```python
from build123d import *

# Parameters (mm, degrees)
SKETCH1_R                 = 31.75
BOSS_EXTRUDE1_DEPTH       = 139
SKETCH3_R                 = 9.5
BOSS_EXTRUDE2_DEPTH       = 2.4
SKETCH3_2_R               = 9.5
BOSS_EXTRUDE3_DEPTH       = 13.75
F_6_32_TAPPED_HOLE1_D     = 2.7051
F_6_32_TAPPED_HOLE1_DEPTH = 9.39
F_6_32_TAPPED_HOLE1_TIP   = 0.81269403
SKETCH7_R                 = 6.25
BOSS_EXTRUDE4_DEPTH       = 2.5
SKETCH7_3_R               = 5
BOSS_EXTRUDE5_DEPTH       = 8.33
SKETCH7_4_R               = 5
BOSS_EXTRUDE6_DEPTH       = 18.5
BOSS_EXTRUDE7_DEPTH       = 0.5


with BuildPart() as part:
    # Sketch1 → Boss-Extrude1 (new, symmetric)
    with BuildSketch(Plane.XY):
        Circle(SKETCH1_R)
    extrude(amount=BOSS_EXTRUDE1_DEPTH, both=True)

    # Sketch3 → Boss-Extrude2 (add)
    with BuildSketch(Plane.XY.offset(139)):
        with BuildLine():
            Line((11.6445, -2.539), (-11.6445, -2.539))
            ThreePointArc((-11.6445, -2.539), (-12.705160172, -2.099660172), (-13.1445, -1.039))
            Line((-13.1445, -1.039), (-13.1445, 22.25))
            ThreePointArc((-13.1445, 22.25), (-12.705160172, 23.310660172), (-11.6445, 23.75))
            Line((-11.6445, 23.75), (11.6445, 23.75))
            ThreePointArc((11.6445, 23.75), (12.705160172, 23.310660172), (13.1445, 22.25))
            Line((13.1445, 22.25), (13.1445, -1.039))
            ThreePointArc((13.1445, -1.039), (12.705160172, -2.099660172), (11.6445, -2.539))
        make_face()
        with Locations((0, 10.6055)):
            Circle(SKETCH3_R, mode=Mode.SUBTRACT)
    extrude(amount=BOSS_EXTRUDE2_DEPTH)

    # Sketch3_2 → Boss-Extrude3 (add)
    with BuildSketch(Plane.XY.offset(139)):
        with Locations((0, 10.6055)):
            Circle(SKETCH3_2_R)
    extrude(amount=BOSS_EXTRUDE3_DEPTH)

    # Sketch4 → Revolve1 (revolve)
    with BuildSketch(Plane(origin=(0, -21.35, 0), x_dir=(1, 0, 0), z_dir=(0, 1, 0))):
        Polygon((0, -139), (0, -143.5), (-0.25, -143.5), (-0.25, -147.5), (-2, -147.5), (-2, -141), (-4.175, -141), (-4.175, -150.5), (-4.75, -150.5), (-4.75, -140), (-5.22, -140), (-5.22, -139), align=None)
    revolve(axis=Axis((0, -21.35, 143.5), (0, 0, 1)))

    # 6-32 Tapped Hole1
    with Locations(Plane.XY.offset(139)):
        with Locations((-20.79625, 0), (20.79625, 0)):
            Hole(F_6_32_TAPPED_HOLE1_D / 2, depth=F_6_32_TAPPED_HOLE1_DEPTH)
            with Locations((0, 0, -(F_6_32_TAPPED_HOLE1_DEPTH + F_6_32_TAPPED_HOLE1_TIP / 2))):  # 118° drill point
                Cone(0, F_6_32_TAPPED_HOLE1_D / 2, F_6_32_TAPPED_HOLE1_TIP, mode=Mode.SUBTRACT)

    # Sketch7 → Boss-Extrude4 (add)
    with BuildSketch(Plane(origin=(0, 0, -139), x_dir=(-1, 0, 0), z_dir=(0, 0, -1))):
        Polygon((29.987604307, 0), (25.368802154, 8), (16.131197846, 8), (11.512395693, 0), (16.131197846, -8), (25.368802154, -8), align=None)
        with Locations((20.75, 0)):
            Circle(SKETCH7_R, mode=Mode.SUBTRACT)
    extrude(amount=BOSS_EXTRUDE4_DEPTH)

    # Sketch7_3 → Boss-Extrude5 (add)
    with BuildSketch(Plane(origin=(0, 0, -139), x_dir=(-1, 0, 0), z_dir=(0, 0, -1))):
        with BuildLine():
            ThreePointArc((27, 0), (19.56140156, 6.135937887), (14.952085201, -2.333813184))
            Line((14.952085201, -2.333813184), (18.416186816, -5.797914799))
            ThreePointArc((18.416186816, -5.797914799), (24.248297271, -5.179229306), (27, 0))
        make_face()
        with Locations((20.75, 0)):
            Circle(SKETCH7_3_R, mode=Mode.SUBTRACT)
    extrude(amount=BOSS_EXTRUDE5_DEPTH)

    # Sketch7_4 → Boss-Extrude6 (add)
    with BuildSketch(Plane(origin=(0, 0, -139), x_dir=(-1, 0, 0), z_dir=(0, 0, -1))):
        with Locations((20.75, 0)):
            Circle(SKETCH7_4_R)
    extrude(amount=BOSS_EXTRUDE6_DEPTH)

    # Sketch8 → Boss-Extrude7 (add)
    with BuildSketch(Plane(origin=(0, 0, -139), x_dir=(-1, 0, 0), z_dir=(0, 0, -1))):
        with BuildLine():
            Line((7.9125, 25.2), (-15.9125, 25.2))
            ThreePointArc((-15.9125, 25.2), (-17.035032015, 24.735032015), (-17.5, 23.6125))
            Line((-17.5, 23.6125), (-17.5, -23.6125))
            ThreePointArc((-17.5, -23.6125), (-17.035032015, -24.735032015), (-15.9125, -25.2))
            Line((-15.9125, -25.2), (7.9125, -25.2))
            ThreePointArc((7.9125, -25.2), (9.035032015, -24.735032015), (9.5, -23.6125))
            Line((9.5, -23.6125), (9.5, 23.6125))
            ThreePointArc((9.5, 23.6125), (9.035032015, 24.735032015), (7.9125, 25.2))
        make_face()
    extrude(amount=BOSS_EXTRUDE7_DEPTH)


solid = part.part
```
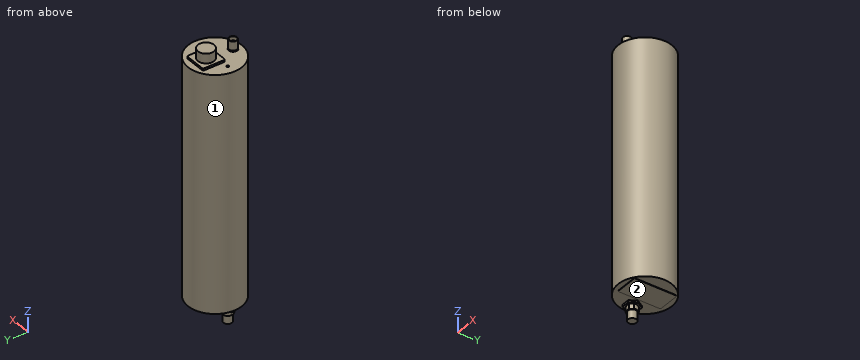
Build history of the part. All positions in model axes, mm. Face numbers are marked on the shaded views. A direction names the side the tool comes from. Round coordinates to 2 decimals unless told otherwise and drop trailing zeros. Loops run counter-clockwise (first coordinate to the right, second up) from the corner with the lowest first, then second, coordinate; pieces in that order, holes last.
Item 1: Pin check, flat tips, straight feed: P1, Ø8, axis at y = -16.5, z = -92.5, coming from the +X side; P2, Ø2, axis at x = 16, z = -106, coming from the -Y side; P3, Ø0.6, axis at y = -11, z = -139, coming from the -X side. Stop position of each tip, or through.
Item 2: Saw through at A-A (y = -11). List the corners of the cut face in (x, z), then the cut area to 3 significant figures.
Item 3: Saw through at B-B (z = -84). List the corners of the cut face in (x, y), then the cut area to 3 significant figures.
Item 4: Which spindle directions (+Z, -Z, +X, -X, +Y, -Y) get a long thin tool onto all of the face, cutting with end or side? Do the marked faces 1 and 2. Say none if no direction does.
Item 5: Drill centre lines: line 1 along X through (y, z) = (-21.35, 146) (3 decimals); line 2 along Z through (x, y) = (-18.5, -24.5); line 3 along Z through (x, y) = (-3, 19). Where is each one in solid material? Low to high.
Worked answers:
1. P1: stops at x = 29.19
1. P2: stops at y = -27.98
1. P3: stops at x = -29.89
2. outline: (-29.78, -139) - (-9.5, -139) - (-9.5, -139.5) - (17.5, -139.5) - (17.5, -139) - (29.78, -139) - (29.78, 139) - (-29.78, 139) - close
2. area: 16,600 mm2
3. outline: circle Ø63.5 at (0, 0)
3. area: 3,170 mm2
4. face 1: +Z, -Z
4. face 2: -Z, +X, +Y, -Y
5. line 1: x = -4.75 to -4.175, -2 to -0.25, 0.25 to 2, 4.175 to 4.75
5. line 2: z = -139 to 139
5. line 3: z = -139.5 to 152.75
